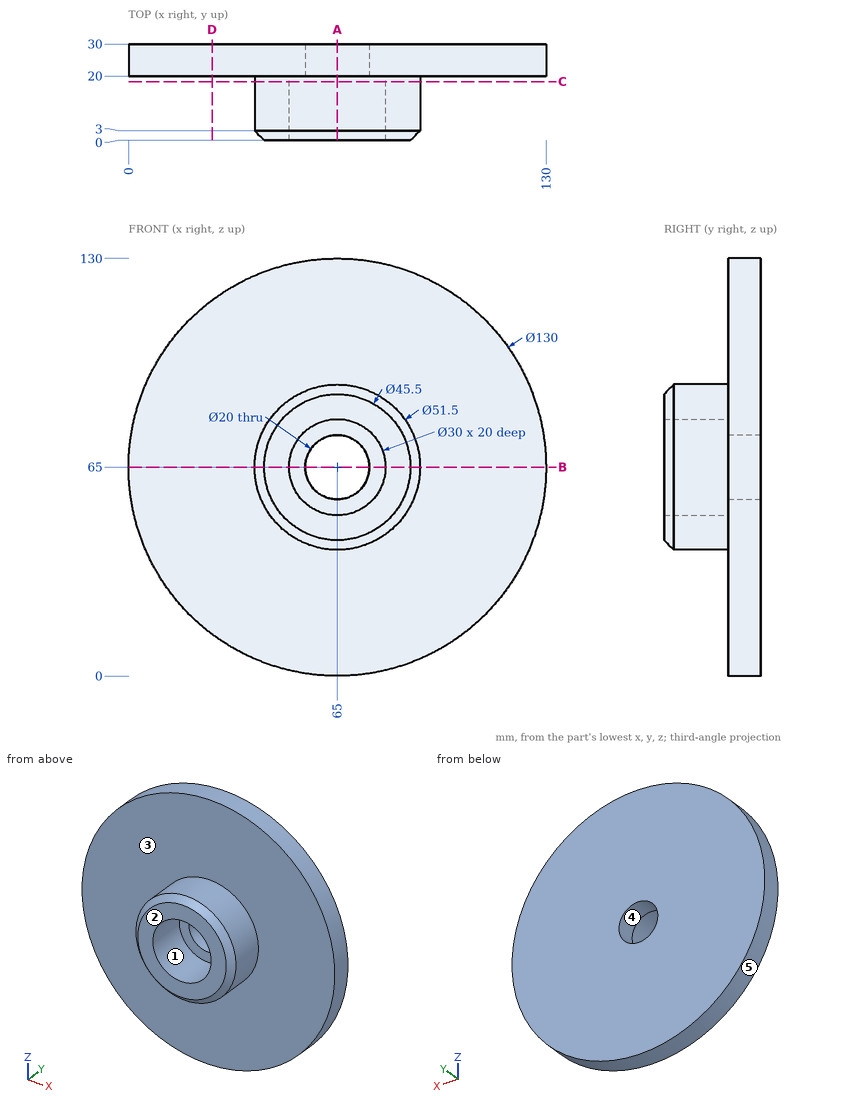
Design review of the part shown in the three views and the two pictorial views. Dimensions are in mm from the part's minimum x, y and z. A direction names the side the tool comes from. Coordinates: 2 decimals unless noted, no trailing zeros. Order: outer loops, then holes, each group sorted by start corner. A loop starts at its lowest first (then second) coordinate and runs counter-clockwise, first axis right, second up. Notation, with made-up numbers: (-25, -6.5) -> (14, -6.5) arc R23 ccw to (14, 17.5) -> close; hole circle Ø1 at (-3.75, -7.5). An arc over 180 degrees is marked (long way). Use one line per item in the form item = value. Start each with the question number.
(1) Add section A-A on x = 65. State the section outline as (y, z) points.
(2) The part is to be moulded in two halves that separate along X. For the marked faces 3, 4 and 5, say which applies: +X half, -X half, draft (parallel to the pull), parting line (faces both ways), or undercut.
(3) Add section B-B on z = 65. State the section outline as (x, y) points.
(4) Add section D-D on x = 26. State the section outline as (y, z) points, plus the area to 3 significant figures.
(5) For the marked faces 1 and 2, list the 3-axis set-ups (+Z, -Z, +X, -X, +Y, -Y) from which the entire face can be reached by the end or side of a thin tool; tool diameter is ignored.
(6) For probe 1 along X at (y, z) = (10, 65); probe 2 along X at (y, z) = (23.25, 65); probe 3 along Z at (x, y) = (70, 4), list the stretches that pass through material, from the lowest coordinate up.
(7) Add section C-C on y = 18.25. State the section outline as (x, z) points.
(8) Insertion check: pin 1 (6 mm diameter, centred on x = 71.5, y = 16.5, fed in from +Z); pin 2 (2 mm diameter, centred on x = 39, y = 26, fed in from +Z); pin 3 (1 mm diameter, centred on x = 31, y = 22, fed in from -Z); pin 4 (12 mm diameter, centred on x = 65, z = 65, fed in from +Y). Each pin has a flat end and moves straight along its axis. Give the tip position at first contact, or say it passes through.
Answer block:
q1.outline = (0, 42.25) -> (3, 39.25) -> (20, 39.25) -> (20, 0) -> (30, 0) -> (30, 55) -> (20, 55) -> (20, 50) -> (0, 50) -> close; (0, 80) -> (20, 80) -> (20, 75) -> (30, 75) -> (30, 130) -> (20, 130) -> (20, 90.75) -> (3, 90.75) -> (0, 87.75) -> close
q2.face_3 = draft
q2.face_4 = undercut
q2.face_5 = parting line
q3.outline = (0, 20) -> (39.25, 20) -> (39.25, 3) -> (42.25, 0) -> (50, 0) -> (50, 20) -> (55, 20) -> (55, 30) -> (0, 30) -> close; (75, 20) -> (80, 20) -> (80, 0) -> (87.75, 0) -> (90.75, 3) -> (90.75, 20) -> (130, 20) -> (130, 30) -> (75, 30) -> close
q4.outline = (20, 13) -> (30, 13) -> (30, 117) -> (20, 117) -> close
q4.area = 1,040 mm²
q5.face_1 = -Y
q5.face_2 = +Z, -Z, +X, -X, -Y
q6.probe_1 = 39.25 to 50, 80 to 90.75
q6.probe_2 = 0 to 55, 75 to 130
q6.probe_3 = 39.74 to 50.86, 79.14 to 90.26
q7.outline = circle Ø51.5 at (65, 65); hole circle Ø30 at (65, 65)
q8.pin_1 = 90.51
q8.pin_2 = 125
q8.pin_3 = 9.3
q8.pin_4 = through
